from build123d import *

# Parameters (mm, degrees)
F0_W     = 187.325
F0_H     = 47.625
F1_DEPTH = 76.2
F2_W     = 187.325
F2_H     = 47.625
F2_W_2   = 168.275
F2_H_2   = 22.225
F3_DEPTH = 4.7625


with BuildPart() as f1:
    # F0 (on Top) → F1 (new body)
    with BuildSketch(Plane.XY):
        with Locations((88.9, 19.05)):
            Rectangle(F0_W, F0_H)
    extrude(amount=-F1_DEPTH)

    # F2 (on face) → F3 (cut)
    with BuildSketch(Plane.XY):
        with Locations((88.9, 19.05)):
            Rectangle(F2_W, F2_H)
        with Locations((88.9, 19.05)):
            Rectangle(F2_W_2, F2_H_2, mode=Mode.SUBTRACT)
    extrude(amount=-F3_DEPTH, mode=Mode.SUBTRACT)


solid = f1.part
Source: CAD feature listing. Evaluate the final solid. Frame: model axes, mm. A direction names the side the tool comes from. Round coordinates to 2 decimals unless told otherwise and drop trailing zeros. Loops run counter-clockwise (first coordinate to the right, second up) from the corner with the lowest first, then second, coordinate; pieces in that order, holes last.
Q1. Section B-B, the plane y = 38. Return loops of the section in (x, z), plus the area to 3 significant figures.
Q2. First-contact query: P1, Ø4, axis at x = 61, y = 11, coming from the +Z side; P2, Ø4, axis at x = 75.5, z = -2.5, coming from the +Y side; P3, Ø4, axis at y = 23, z = -2, coming from the -X side; P4, Ø1.4, axis at y = 21.5, z = -2, coming from the +X side. Flat tips, straight axial feed; report the tip coordinate or a pass-through.
Q3. Ray query, line 1 (Z direction, x = 127, y = 0); line 2 (Y direction, x = 50, z = -3). Return the intervals inside material, ascending.
Q4. Section A-A, the plane x = 24. Return loops of the section in (y, z), plus the area to 3 significant figures.
Q5. Access query for faces 1 (the face through (173.038, 19, -2)), 2 (the face through (88, 30.162, -2)), 3 (the face through (88, 7.938, -2)). Directions: +Z, -Z, +X, -X, +Y, -Y. A direction counts if a zero-diameter tool reaches every point of the face in a straight line with its end or side. Return the directions, or none.
Solutions:
1. outline: (-4.76, -76.2) - (182.56, -76.2) - (182.56, -4.76) - (-4.76, -4.76) - close
1. area: 13,400 mm2
2. P1: stops at z = 0
2. P2: stops at y = 30.16
2. P3: stops at x = 4.76
2. P4: stops at x = 173.04
3. line 1: z = -76.2 to -4.76
3. line 2: y = 7.94 to 30.16
4. outline: (-4.76, -76.2) - (42.86, -76.2) - (42.86, -4.76) - (30.16, -4.76) - (30.16, 0) - (7.94, 0) - (7.94, -4.76) - (-4.76, -4.76) - close
4. area: 3,510 mm2
5. face 1: +Z, +X, +Y, -Y
5. face 2: +Z, +X, -X, +Y
5. face 3: +Z, +X, -X, -Y
